```python
from build123d import *

# Parameters (mm, degrees)
F0_W      = 45
F0_H      = 45
F1_DEPTH  = 30
F2_SIZE   = 3
F4_D      = 5
F6_DEPTH  = 20
F7_R      = 9
F8_DEPTH  = 5
F10_D     = 10
F10_DEPTH = 30
F10_TIP   = 3.0043030951
F11_R     = 20
F12_DEPTH = 5


with BuildPart() as f1:
    # F0 (on Top) → F1 (new body)
    with BuildSketch(Plane.XY):
        with Locations((-22.5, -22.5)):
            Rectangle(F0_W, F0_H)
    extrude(amount=F1_DEPTH)

    # F2
    f2_edges = [f1.edges().sort_by_distance(p)[0] for p in [
        (-45, -45, 15),
        (0, -45, 15),
        (0, 0, 15),
        (-45, 0, 15),
    ]]
    chamfer(f2_edges, length=F2_SIZE)

    # F4 (through all)
    with Locations(Plane.XY.offset(30)):
        with Locations((-40.5312229203, -40.5312229203), (-40.5312229203, -4.4687770797), (-4.4687770797, -4.4687770797), (-4.4687770797, -40.5312229203)):
            Hole(F4_D / 2)

    # F5 (on face) → F6 (join)
    with BuildSketch(Plane.YZ):
        with BuildLine():
            ThreePointArc((-15.3121332332, 12.8588387864), (-15.0784435342, 13.9181036905), (-15, 15))
            ThreePointArc((-15, 15), (-15.2293520832, 16.8405648237), (-15.903381032, 18.5685596803))
            ThreePointArc((-15.903381032, 18.5685596803), (-17.7711474831, 20.8213360901), (-20.3588389028, 22.1878668015))
            ThreePointArc((-20.3588389028, 22.1878668015), (-23.2725024385, 22.4601099176), (-26.0685594955, 21.5966190679))
            ThreePointArc((-26.0685594955, 21.5966190679), (-28.3213359619, 19.7288526747), (-29.6878667454, 17.1411612856))
            ThreePointArc((-29.6878667454, 17.1411612856), (-29.9601099219, 14.2274976035), (-29.0966190145, 11.4314404058))
            ThreePointArc((-29.0966190145, 11.4314404058), (-27.2288526423, 9.1786640118), (-24.6411613131, 7.8121332628))
            ThreePointArc((-24.6411613131, 7.8121332628), (-21.7274976178, 7.5398900766), (-18.9314404058, 8.4033809855))
            ThreePointArc((-18.9314404058, 8.4033809855), (-16.6786639791, 10.271147398), (-15.3121332332, 12.8588387864))
        make_face()
        with BuildLine():
            ThreePointArc((-15.903381032, 18.5685596803), (-15.2293520832, 16.8405648237), (-15, 15))
            ThreePointArc((-15, 15), (-15.0784435342, 13.9181036905), (-15.3121332332, 12.8588387864))
            Line((-15.3121332332, 12.8588387864), (-14.4252352272, 15.8361507619))
            Line((-14.4252352272, 15.8361507619), (-15.903381032, 18.5685596803))
        make_face()
        with BuildLine():
            ThreePointArc((-20.3588389028, 22.1878668015), (-17.7711474831, 20.8213360901), (-15.903381032, 18.5685596803))
            Line((-15.903381032, 18.5685596803), (-17.3815269465, 21.3009688012))
            Line((-17.3815269465, 21.3009688012), (-20.3588389028, 22.1878668015))
        make_face()
        with BuildLine():
            Line((-16.1990311988, 9.8815269465), (-15.3121332332, 12.8588387864))
            ThreePointArc((-15.3121332332, 12.8588387864), (-16.6786639791, 10.271147398), (-18.9314404058, 8.4033809855))
            Line((-18.9314404058, 8.4033809855), (-16.1990311988, 9.8815269465))
        make_face()
        with BuildLine():
            ThreePointArc((-26.0685594955, 21.5966190679), (-23.2725024385, 22.4601099176), (-20.3588389028, 22.1878668015))
            Line((-20.3588389028, 22.1878668015), (-23.3361507619, 23.0747647728))
            Line((-23.3361507619, 23.0747647728), (-26.0685594955, 21.5966190679))
        make_face()
        with BuildLine():
            Line((-21.6638492381, 6.9252352272), (-18.9314404058, 8.4033809855))
            ThreePointArc((-18.9314404058, 8.4033809855), (-21.7274976178, 7.5398900766), (-24.6411613131, 7.8121332628))
            Line((-24.6411613131, 7.8121332628), (-21.6638492381, 6.9252352272))
        make_face()
        with BuildLine():
            ThreePointArc((-29.6878667454, 17.1411612856), (-28.3213359619, 19.7288526747), (-26.0685594955, 21.5966190679))
            Line((-26.0685594955, 21.5966190679), (-28.8009688012, 20.1184730535))
            Line((-28.8009688012, 20.1184730535), (-29.6878667454, 17.1411612856))
        make_face()
        with BuildLine():
            Line((-27.6184730535, 8.6990311988), (-24.6411613131, 7.8121332628))
            ThreePointArc((-24.6411613131, 7.8121332628), (-27.2288526423, 9.1786640118), (-29.0966190145, 11.4314404058))
            Line((-29.0966190145, 11.4314404058), (-27.6184730535, 8.6990311988))
        make_face()
        with BuildLine():
            ThreePointArc((-29.0966190145, 11.4314404058), (-29.9601099219, 14.2274976035), (-29.6878667454, 17.1411612856))
            Line((-29.6878667454, 17.1411612856), (-30.5747647728, 14.1638492381))
            Line((-30.5747647728, 14.1638492381), (-29.0966190145, 11.4314404058))
        make_face()
    extrude(amount=F6_DEPTH)

    # F7 (on face) → F8 (join)
    with BuildSketch(Plane.YZ.offset(20)):
        with Locations((-22.5, 15)):
            Circle(F7_R)
        Polygon((-29.687866787, 17.1411611458), (-22.5, 15), (-24.6411611458, 7.812133213), align=None, mode=Mode.SUBTRACT)
        Polygon((-24.6411611458, 7.812133213), (-22.5, 15), (-29.687866787, 17.1411611458), align=None)
    extrude(amount=F8_DEPTH)

    # F10
    with Locations(Plane.YZ.offset(25)):
        with Locations((-22.5, 15)):
            Hole(F10_D / 2, depth=F10_DEPTH)
            with Locations((0, 0, -(F10_DEPTH + F10_TIP / 2))):  # 118° drill point
                Cone(0, F10_D / 2, F10_TIP, mode=Mode.SUBTRACT)

    # F11 (on face) → F12 (cut)
    with BuildSketch(Plane.XY.offset(30)):
        with Locations((-22.5, -22.5)):
            Circle(F11_R)
    extrude(amount=-F12_DEPTH, mode=Mode.SUBTRACT)


solid = f1.part
```
Here's how the part is built. I have some questions about the finished solid (model axes, mm). A direction names the side the tool comes from. Coordinates: 2 decimals unless noted, no trailing zeros. Write each loop counter-clockwise with the first axis right and the second up, starting at its lowest first coordinate (ties: lowest second). Pieces come first, ordered by that corner, then holes. Notation, with made-up numbers: (49, 31) -> (104, 31) arc R30 cw to (104, 65) -> close; hole circle Ø5 at (58.25, 25.5). An arc over 180 degrees is marked (long way). Use a Markdown table: item, result. Add a question column.
(1) Please list where these lines run through material, in increasing order: line 1 (Y direction, x = -4.5, z = 6.5); line 2 (Y direction, x = -22.5, z = 27.1); line 3 (Y direction, x = -42, z = 17).
(2) If we section it at C-C, the plane z = 3: Write out the boundary of the cut face in (x, y).
(3) If we section it at B-B, the plane y = -39: Write out the boundary of the cut face in (x, z).
(4) If we section it at A-A, the plane x = 7.5: Write out the boundary of the cut face in (y, z), and give its area (3 significant figures).
(5) We'd pull the mould along Z, two halves only. Please class faces 4 (the cylindrical face through (-42.84, -41.49, 14.79)), 5 (the conical face through (-7.483, -22.613, 15.861)), 6 (the cylindrical face through (22.465, -13.916, 17.703)): +Z half, -Z half, draft (parallel to the pull), parting line (faces both ways), or undercut.
(6) For faces 1 (the flat face through (-23, -22, 25)), 2 (the flat face through (9.86, -29.117, 11.47)), 3 (the cylindrical face through (9.79, -21.42, 10.12)), which set-ups out of +Z, -Z, +X, -X, +Y, -Y let a thin tool reach every point of the face, with its end or its side?
(7) I'm going to push flat-ended pins straight in: P1, Ø4.5, axis at x = -40.53, y = -40.53, coming from the +Z side (3 decimals); P2, Ø2, axis at y = -35.5, z = 16, coming from the +X side; P3, Ø20, axis at x = -18.5, y = -20.5, coming from the +Z side; P4, Ø12, axis at x = 9.5, y = -34.5, coming from the +Z side. Where does each tip first touch, or does it pass through?
(8) If we section it at D-D, the plane x = -33: Write out the boundary of the cut face in (y, z).
Outcome:
| question | item | result |
|---|---|---|
| 1 | line 1 | y = -45 to -43.03, -38.03 to -6.97, -1.97 to 0 |
| 1 | line 2 | y = -45 to -42.5, -2.5 to 0 |
| 1 | line 3 | y = -45 to -42.55, -38.51 to -6.49, -2.45 to 0 |
| 2 | outline | (-45, -42) -> (-42, -45) -> (-3, -45) -> (0, -42) -> (0, -3) -> (-3, 0) -> (-42, 0) -> (-45, -3) -> close; hole circle Ø5 at (-40.53, -40.53); hole circle Ø5 at (-40.53, -4.47); hole circle Ø5 at (-4.47, -40.53); hole circle Ø5 at (-4.47, -4.47) |
| 3 | outline | (-45, 0) -> (-42.51, 0) -> (-42.51, 30) -> (-45, 30) -> close; (-38.56, 0) -> (-6.44, 0) -> (-6.44, 30) -> (-11.2, 30) -> (-11.2, 25) -> (-33.8, 25) -> (-33.8, 30) -> (-38.56, 30) -> close; (-2.49, 0) -> (0, 0) -> (0, 30) -> (-2.49, 30) -> close |
| 4 | outline | (-30.57, 14.16) -> (-27.62, 8.7) -> (-21.66, 6.93) -> (-16.2, 9.88) -> (-14.43, 15.84) -> (-17.38, 21.3) -> (-23.34, 23.07) -> (-28.8, 20.12) -> close; hole circle Ø10 at (-22.5, 15) |
| 4 | area | 108 mm^2 |
| 5 | face 4 | draft |
| 5 | face 5 | undercut |
| 5 | face 6 | parting line |
| 6 | face 1 | +Z |
| 6 | face 2 | -Z, -Y |
| 6 | face 3 | +X |
| 7 | P1 | passes through |
| 7 | P2 | stops at x = 0 |
| 7 | P3 | stops at z = 25 |
| 7 | P4 | stops at z = 20.28 |
| 8 | outline | (-45, 0) -> (0, 0) -> (0, 30) -> (-5.48, 30) -> (-5.48, 25) -> (-39.52, 25) -> (-39.52, 30) -> (-45, 30) -> close |
